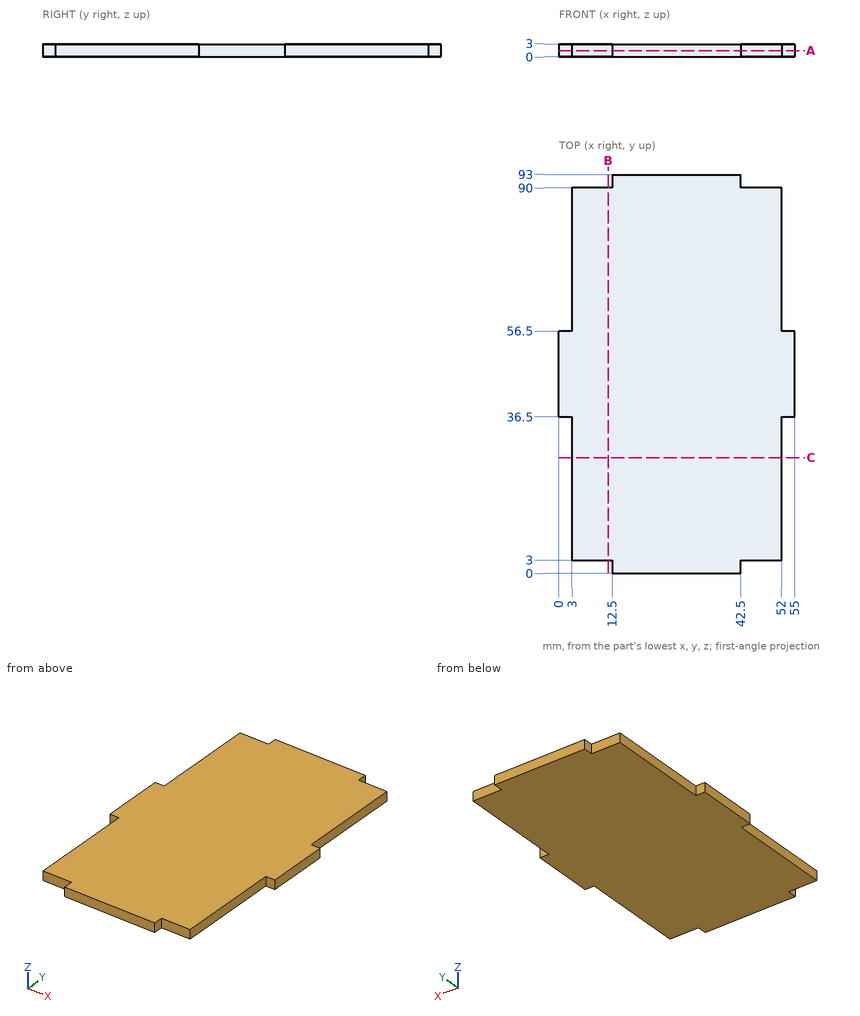
Can you work these out from the drawing? Everything is in mm from the part's minimum corner. Give positions to 0.01 mm unless a question says otherwise; leave off trailing zeros. Write each loop counter-clockwise with the first axis right and the second up, starting at its lowest first coordinate (ties: lowest second). Pieces come first, ordered by that corner, then holes. Notation, with made-up numbers: M 19.5,52 L 50.5,52 A29 cw 50.5,88 Z; hole C -10,-37 d8. An arc over 180 degrees is marked long. Answer in a Markdown table with one row per item. Add a question column.
Item 1: Imagine slicing it at B-B, the plane x = 11.5. Write out the boundary of the cut face in (y, z), plus the area to 3 significant figures.
Item 2: Please list where these lines run through material, in increasing order: L1, parallel to Y at x = 51, z = 2.2; L2, parallel to X at y = 87.5, z = 0.3.
Item 3: Imagine slicing it at A-A, the plane z = 1.45. Write out the boundary of the cut face in (x, y).
Item 4: For pin 1 Ø1.5 at (y, z) = (92, 2) entering from -X; pin 2 Ø0.9 at (x, z) = (45.5, 1) entering from -Y; pin 3 Ø1.5 at (y, z) = (91.5, 1.5) entering from +X; pin 4 Ø3 at (x, y) = (38, 13) entering from -Z, each with a flat end and sliding along its axis, tell me the tip position at first contact or that it passes through.
Item 5: Imagine slicing it at C-C, the plane y = 27. Write out the boundary of the cut face in (x, z), plus the area to 3 significant figures.
Evaluation:
| question | item | result |
|---|---|---|
| 1 | outline | M 3,0 L 90,0 L 90,3 L 3,3 Z |
| 1 | area | 261 mm² |
| 2 | L1 | y = 3 to 90 |
| 2 | L2 | x = 3 to 52 |
| 3 | outline | M 0,36.5 L 3,36.5 L 3,3 L 12.5,3 L 12.5,0 L 42.5,0 L 42.5,3 L 52,3 L 52,36.5 L 55,36.5 L 55,56.5 L 52,56.5 L 52,90 L 42.5,90 L 42.5,93 L 12.5,93 L 12.5,90 L 3,90 L 3,56.5 L 0,56.5 Z |
| 4 | pin 1 | stops at x = 12.5 |
| 4 | pin 2 | stops at y = 3 |
| 4 | pin 3 | stops at x = 42.5 |
| 4 | pin 4 | stops at z = 0 |
| 5 | outline | M 3,0 L 52,0 L 52,3 L 3,3 Z |
| 5 | area | 147 mm² |
